Autodesk Inventor part; units mm, degrees
ref_plane "YZ Plane" through (0, 0, 0) normal (1, 0, 0) x (0, 1, 0)
ref_plane "XZ Plane" through (0, 0, 0) normal (0, 1, 0) x (-1, 0, 0)
ref_plane "XY Plane" through (0, 0, 0) normal (0, 0, 1) x (1, 0, 0)
sketch "Sketch1" plane through (0, 0, 0) normal (0, 0, 1) x (1, 0, 0)
  line L0 (-3.3239, 4.8371) -> (16.6761, 4.8371)
  line L1 (16.6761, 4.8371) -> (16.6761, -15.1629)
  line L2 (16.6761, -15.1629) -> (-3.3239, -15.1629)
  line L3 (-3.3239, -15.1629) -> (-3.3239, 4.8371)
  line L4 (14.5634, -0.1629) -> (29.6761, -0.1629)
  line L5 (29.6761, -0.1629) -> (29.6761, -10.1629)
  line L6 (29.6761, -10.1629) -> (14.5634, -10.1629)
  line L7 (14.5634, -10.1629) -> (14.5634, -0.1629)
  line L8 (-1.0107, -0.1629) -> (-16.3239, -0.1629)
  line L9 (-16.3239, -0.1629) -> (-16.3239, -10.1629)
  line L10 (-16.3239, -10.1629) -> (-1.0107, -10.1629)
  line L11 (-1.0107, -10.1629) -> (-1.0107, -0.1629)
  line L12 (-3.3239, 4.8371) -> (-8.3239, -0.1629)
  line L13 (16.6761, 4.8371) -> (21.6761, -0.1629)
  line L14 (-3.3239, -15.1629) -> (-8.3239, -10.1629)
  line L15 (16.6761, -15.1629) -> (21.6761, -10.1629)
  point P0 (0, 0)
  dimension "d0" = 20
  dimension "d1" = 20
  dimension "d2" = 10
  dimension "d3" = 10
  dimension "d4" = 0
  dimension "d5" = 5
  dimension "d6" = 13
  dimension "d7" = 13
  dimension "d10" = 45
  dimension "d11" = 45
  dimension "d12" = 45
extrude "Extrusion1" add sketch "Sketch1" along normal blind 6.35
properties part number "ColdFingerStem"
Here's how the part is built. I have some questions about the finished solid (model axes, mm). A direction names the side the tool comes from. Give positions to 0.01 mm unless a question says otherwise; leave off trailing zeros. Write each loop counter-clockwise with the first axis right and the second up, starting at its lowest first coordinate (ties: lowest second). Pieces come first, ordered by that corner, then holes.
(1) On a 3-axis mill with a long thin cutter (end or side, diameter ignored), from which of +Z, -Z, +X, -X, +Y, -Y can I reach the whole of each face in a straight line? I mean faces 1 (the face through (-12, -10.163, 3)), 2 (the face through (26, -0.163, 3)), 3 (the face through (26, -10.163, 3)). Say none if no direction works.
Output values:
face 1: +Z, -Z, -X, -Y
face 2: +Z, -Z, +X, +Y
face 3: +Z, -Z, +X, -Y
(2) Will these pins go through, and if not, where does the flat tip stop? pin 1 (1.9 mm diameter, centred on x = 24.5, z = 2.5, fed in from +Y); pin 2 (1.9 mm diameter, centred on x = -11, z = 2.5, fed in from -Y).
Output values:
pin 1: stops at y = -0.16
pin 2: stops at y = -10.16
(3) Imagine slicing it at A-A, the plane z = 3.5. Write out the boundary of the cut face in (x, y).
Output values:
outline: (-16.32, -10.16) - (-8.32, -10.16) - (-3.32, -15.16) - (16.68, -15.16) - (21.68, -10.16) - (29.68, -10.16) - (29.68, -0.16) - (21.68, -0.16) - (16.68, 4.84) - (-3.32, 4.84) - (-8.32, -0.16) - (-16.32, -0.16) - close
(4) If I drill on L1, parallel to Y at x = 25.5, z = 1.25; L2, parallel to X at y = 4, z = 3.5; L3, parallel to X at y = -14, z = 3.75, over which ranges is the centre line in solid material (lowest first)?
Output values:
L1: y = -10.16 to -0.16
L2: x = -4.16 to 17.51
L3: x = -4.49 to 17.84
(5) Imagine slicing it at C-C, the plane y = -14. Write out the boundary of the cut face in (x, z), and give its area (3 significant figures).
Output values:
outline: (-4.49, 0) - (17.84, 0) - (17.84, 6.35) - (-4.49, 6.35) - close
area: 142 mm2
(6) Imagine slicing it at B-B, the plane x = 23. Write out the boundary of the cut face in (y, z), and give its area (3 significant figures).
Output values:
outline: (-10.16, 0) - (-0.16, 0) - (-0.16, 6.35) - (-10.16, 6.35) - close
area: 63.5 mm2
